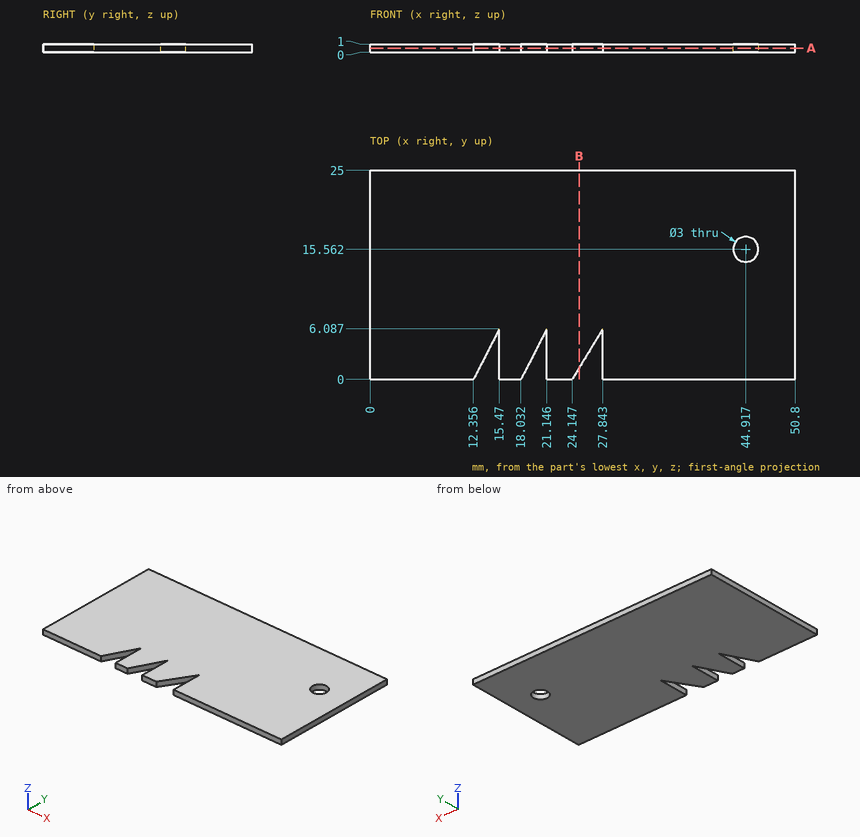
For this review, use the dimensioned drawing (mm, ordinates from the lowest corner) and the shaded views. Coordinates: 2 decimals unless noted, no trailing zeros. Loops run counter-clockwise (first coordinate to the right, second up) from the corner with the lowest first, then second, coordinate; pieces in that order, holes last. Notation, with made-up numbers: (-25.75, -13) - (-15.75, -13) arc R19 ccw to (-15.75, -8) - close; hole circle Ø8 at (-39, 2). An arc over 180 degrees is marked (long way). Use CSV: the item, a comma, the result in double quotes. Start each with the question number.
1) Consider section A-A on z = 0.5. Write out the cut boundary in (x, y).
2) Wall thickness on L1, parallel to X at y = 3.25, z = 0.25 (1 decimal); L2, parallel to X at y = 3.5, z = 0.7 (1 decimal); L3, parallel to Y at x = 44.5, z = 0.8: over which ranges is each line inside the solid? List them lowest first. Write a range as from..to.
3) Consider section B-B on x = 25. Write out the cut boundary in (y, z) (1 decimal).
Geometry says:
1,outline,"(0, 0) - (12.36, 0) - (15.47, 6.09) - (15.47, 0) - (18.03, 0) - (21.15, 6.09) - (21.15, 0) - (24.15, 0) - (27.84, 6.09) - (27.84, 0) - (50.8, 0) - (50.8, 25) - (0, 25) - close; hole circle Ø3 at (44.92, 15.56)"
2,L1,"0..14, 15.5..19.7, 21.1..26.1, 27.8..50.8"
2,L2,"0..14.1, 15.5..19.8, 21.1..26.3, 27.8..50.8"
2,L3,"0..14.12, 17..25"
3,outline,"(1.4, 0) - (25, 0) - (25, 1) - (1.4, 1) - close"
